```python
from build123d import *

# Parameters (mm, degrees)
SKETCH_W        = 22.8
SKETCH_H        = 9
PAD_DEPTH       = 28
FILLET_R        = 1
FILLET001_R     = 1
SKETCH001_W     = 27.634385
SKETCH001_H     = 5
POCKET_DEPTH    = 23.5
SKETCH002_R     = 0.75
POCKET001_DEPTH = 30
SKETCH003_R     = 1.6
POCKET002_DEPTH = 20
CHAMFER_SIZE    = 2
CHAMFER001_SIZE = 2


with BuildPart() as part:
    # Sketch → Pad (new body)
    with BuildSketch(Plane.XY):
        Rectangle(SKETCH_W, SKETCH_H)
    extrude(amount=PAD_DEPTH)

    # Fillet
    fillet_edges = [part.edges().sort_by_distance(p)[0] for p in [
        (11.4, 0, 28),
    ]]
    fillet(fillet_edges, radius=FILLET_R)

    # Fillet001
    fillet001_edges = [part.edges().sort_by_distance(p)[0] for p in [
        (-11.4, 0, 28),
    ]]
    fillet(fillet001_edges, radius=FILLET001_R)

    # Sketch001 (on Face2 of Fillet001) → Pocket (cut)
    with BuildSketch(Plane.XY.offset(28)):
        with Locations((-0.375196, 0)):
            Rectangle(SKETCH001_W, SKETCH001_H)
    extrude(amount=-POCKET_DEPTH, mode=Mode.SUBTRACT)

    # Sketch002 (on Face6 of Pocket) → Pocket001 (cut)
    with BuildSketch(Plane.YZ.offset(11.4)):
        with Locations((0, 2)):
            Circle(SKETCH002_R)
    extrude(amount=-POCKET001_DEPTH, mode=Mode.SUBTRACT)

    # Sketch003 (on Face1 of Pocket) → Pocket002 (cut)
    with BuildSketch(Plane(origin=(0, 4.5, 0), x_dir=(-1, 0, 0), z_dir=(0, 1, 0))):
        with Locations((-6.4, 21)):
            Circle(SKETCH003_R)
        with Locations((6.4, 21)):
            Circle(SKETCH003_R)
    extrude(amount=-POCKET002_DEPTH, mode=Mode.SUBTRACT)

    # Chamfer
    chamfer_edges = [part.edges().sort_by_distance(p)[0] for p in [
        (0, -4.5, 0),
    ]]
    chamfer(chamfer_edges, length=CHAMFER_SIZE)

    # Chamfer001
    chamfer001_edges = [part.edges().sort_by_distance(p)[0] for p in [
        (0, 4.5, 0),
    ]]
    chamfer(chamfer001_edges, length=CHAMFER001_SIZE)


solid = part.part
```
Read the model definition and answer for the solid it produces. Units are mm, in the model's axes. A direction names the side the tool comes from. Coordinates: 2 decimals unless noted, no trailing zeros. Write each loop counter-clockwise with the first axis right and the second up, starting at its lowest first coordinate (ties: lowest second). Pieces come first, ordered by that corner, then holes. Notation, with made-up numbers: (28.5, 3.5) - (86.5, 3.5) arc R7 ccw to (86.5, 9.5) - close; hole circle Ø10 at (14.5, 67). An arc over 180 degrees is marked (long way). Answer as a JSON object with one key per item and string values. Group by question number.
1. Which of the six approach directions +Z, -Z, +X, -X, +Y, -Y give full straight-line access (tool end or side, diameter ignored) to faces 4 (the flat face through (0, -2.5, 16)), 5 (the flat face through (11.4, -3, 10))?
2. The mould has two halves that part along X. Classify faces 1 (the flat face through (0, 2.5, 16)), 2 (the flat face through (-11.4, -3, 10)), 3 (the cylindrical face through (6.608, -3.486, 22.586)): +X half, -X half, draft (parallel to the pull), parting line (faces both ways), or undercut.
3. A cutting plane is placed at B-B (z = 21). Determine the outline of the cut face in (x, y).
4. A cutting plane is placed at C-C (y = 0). Determine the outline of the cut face in (x, z), plus the area to 3 significant figures.
5. A cutting plane is placed at A-A (x = 6.4). Determine the outline of the cut face in (y, z).
6. Consider L1, parallel to Y at x = 7.5, z = 9; L2, parallel to Z at x = -6.5, y = 0; L3, parallel to Z at x = -3, y = 1.5. Determine where each line is inside the solid, lowest interval first. Write a range as [from, to].
7. A cutting plane is placed at D-D (z = 6). Determine the outline of the cut face in (x, y), plus the area to 3 significant figures.
8. This flat-tipped pin is pushed along its axis until it touches: P1, Ø1.9, axis at x = 6.4, z = 21, coming from the +Y side. Where does it stop, or does it pass through?
Worked out:
{
 "1": {"face 4": "+Z, +X, -X", "face 5": "+Z, -Z, +X, +Y, -Y"},
 "2": {"face 1": "draft", "face 2": "-X half", "face 3": "undercut"},
 "3": {"outline": "(-11.4, -4.5) - (-8, -4.5) - (-8, -2.5) - (-11.4, -2.5) - close; (-11.4, 2.5) - (-8, 2.5) - (-8, 4.5) - (-11.4, 4.5) - close; (-4.8, -4.5) - (4.8, -4.5) - (4.8, -2.5) - (-4.8, -2.5) - close; (-4.8, 2.5) - (4.8, 2.5) - (4.8, 4.5) - (-4.8, 4.5) - close; (8, -4.5) - (11.4, -4.5) - (11.4, -2.5) - (8, -2.5) - close; (8, 2.5) - (11.4, 2.5) - (11.4, 4.5) - (8, 4.5) - close"},
 "4": {"outline": "(-11.4, 0) - (11.4, 0) - (11.4, 1.25) - (-11.4, 1.25) - close; (-11.4, 2.75) - (11.4, 2.75) - (11.4, 4.5) - (-11.4, 4.5) - close", "area": "68.4 mm²"},
 "5": {"outline": "(-4.5, 2) - (-2.5, 0) - (2.5, 0) - (4.5, 2) - (4.5, 19.4) - (2.5, 19.4) - (2.5, 4.5) - (-2.5, 4.5) - (-2.5, 19.4) - (-4.5, 19.4) - close; (-4.5, 22.6) - (-2.5, 22.6) - (-2.5, 28) - (-4.5, 28) - close; (2.5, 22.6) - (4.5, 22.6) - (4.5, 28) - (2.5, 28) - close; hole circle Ø1.5 at (0, 2)"},
 "6": {"L1": "y = [-4.5, -2.5], [2.5, 4.5]", "L2": "z = [0, 1.25], [2.75, 4.5]", "L3": "z = [0, 4.5]"},
 "7": {"outline": "(-11.4, -4.5) - (11.4, -4.5) - (11.4, -2.5) - (-11.4, -2.5) - close; (-11.4, 2.5) - (11.4, 2.5) - (11.4, 4.5) - (-11.4, 4.5) - close", "area": "91.2 mm²"},
 "8": {"P1": "passes through"}
}
